```python
from build123d import *

# Parameters (mm, degrees)
SKETCH_R           = 62.5
SKETCH_R_2         = 7.75
SKETCH_R_3         = 1.5
SKETCH_R_4         = 5.5
SKETCH_R_5         = 4
PAD_DEPTH          = 10
SKETCH001_R        = 11.75
POCKET_DEPTH       = 3
FILLET_R           = 5
FILLET_FACE6_W     = 5
FILLET_FACE6_H     = 10
POCKET001_DEPTH    = 7
POCKET001_FACE39_W = 50
POCKET001_FACE39_H = 10
POCKET002_DEPTH    = 40.001
SKETCH002_R        = 1.5
POCKET003_DEPTH    = 10.001
POCKET004_DEPTH    = 10.001
CHAMFER_SIZE2      = 15
CHAMFER_SIZE       = 8.99
FILLET001_R        = 5


with BuildPart() as part:
    # Sketch → Pad (new body)
    with BuildSketch(Plane.XY):
        Polygon((-100, 100.02), (-100, -99.98), (55, -99.98), (55, -56.98), (60, -56.98), (60, -99.98), (100, -99.98), (100, 100.02), align=None)
        Circle(SKETCH_R, mode=Mode.SUBTRACT)
        with Locations((-82.5, -82.48)):
            Circle(SKETCH_R_2, mode=Mode.SUBTRACT)
        with Locations((-95, -94.98)):
            Circle(SKETCH_R_3, mode=Mode.SUBTRACT)
        with Locations((-95, -69.98)):
            Circle(SKETCH_R_3, mode=Mode.SUBTRACT)
        with Locations((-70, -69.98)):
            Circle(SKETCH_R_3, mode=Mode.SUBTRACT)
        with Locations((-70, -94.98)):
            Circle(SKETCH_R_3, mode=Mode.SUBTRACT)
        with Locations((-95, 95.02)):
            Circle(SKETCH_R_3, mode=Mode.SUBTRACT)
        with Locations((-70, 95.02)):
            Circle(SKETCH_R_3, mode=Mode.SUBTRACT)
        with Locations((-70, 70.02)):
            Circle(SKETCH_R_3, mode=Mode.SUBTRACT)
        with Locations((-95, 70.02)):
            Circle(SKETCH_R_3, mode=Mode.SUBTRACT)
        with Locations((-82.5, 82.52)):
            Circle(SKETCH_R_2, mode=Mode.SUBTRACT)
        with Locations((82.5, 82.52)):
            Circle(SKETCH_R_2, mode=Mode.SUBTRACT)
        with Locations((70, 95.02)):
            Circle(SKETCH_R_3, mode=Mode.SUBTRACT)
        with Locations((95, 95.02)):
            Circle(SKETCH_R_3, mode=Mode.SUBTRACT)
        with Locations((95, 70.02)):
            Circle(SKETCH_R_3, mode=Mode.SUBTRACT)
        with Locations((70, 70.02)):
            Circle(SKETCH_R_3, mode=Mode.SUBTRACT)
        with Locations((-85.5, 0)):
            Circle(SKETCH_R_4, mode=Mode.SUBTRACT)
        with Locations((-85.5, 8)):
            Circle(SKETCH_R_3, mode=Mode.SUBTRACT)
        with Locations((-77.5, 0)):
            Circle(SKETCH_R_3, mode=Mode.SUBTRACT)
        with Locations((-85.5, -8)):
            Circle(SKETCH_R_3, mode=Mode.SUBTRACT)
        with Locations((-93.5, 0)):
            Circle(SKETCH_R_3, mode=Mode.SUBTRACT)
        with Locations((0, 74.23)):
            Circle(SKETCH_R_5, mode=Mode.SUBTRACT)
        with Locations((68, -94.98)):
            Circle(SKETCH_R_3, mode=Mode.SUBTRACT)
        with Locations((93, -94.98)):
            Circle(SKETCH_R_3, mode=Mode.SUBTRACT)
    extrude(amount=PAD_DEPTH)

    # Sketch001 (on Face34 of Pad) → Pocket (cut)
    with BuildSketch(Plane.XY.offset(10)):
        with Locations((-85.5, 0)):
            Circle(SKETCH001_R)
    extrude(amount=-POCKET_DEPTH, mode=Mode.SUBTRACT)

    # Fillet
    fillet_edges = [part.edges().sort_by_distance(p)[0] for p in [
        (-100, -99.98, 5),
        (-100, 100.02, 5),
        (100, 100.02, 5),
        (100, -99.98, 5),
    ]]
    fillet(fillet_edges, radius=FILLET_R)

    # Fillet Face6 → Pocket001 (cut)
    with BuildSketch(Plane(origin=(57.5, -56.98, 5), x_dir=(-1, 0, 0), z_dir=(0, -1, 0))):
        Rectangle(FILLET_FACE6_W, FILLET_FACE6_H)
    extrude(amount=-POCKET001_DEPTH, mode=Mode.SUBTRACT)

    # Pocket001 Face39 → Pocket002 (cut, through all)
    with BuildSketch(Plane(origin=(60, -74.98, 5), x_dir=(0, 1, 0), z_dir=(-1, 0, 0))):
        Rectangle(POCKET001_FACE39_W, POCKET001_FACE39_H)
    extrude(amount=-POCKET002_DEPTH, mode=Mode.SUBTRACT)

    # Sketch002 (on Face32 of Pocket002) → Pocket003 (cut, through all)
    with BuildSketch(Plane.XY.offset(10)):
        with Locations((62.5, -45)):
            Circle(SKETCH002_R)
        with Locations((92.5, -45)):
            Circle(SKETCH002_R)
    extrude(amount=-POCKET003_DEPTH, mode=Mode.SUBTRACT)

    # Sketch003 (on Face35 of Pocket003) → Pocket004 (cut, through all)
    with BuildSketch(Plane.XY.offset(10)):
        Polygon((55, -58), (48, -58), (48, -67), (20, -67), (20, -100), (55, -100), align=None)
    extrude(amount=-POCKET004_DEPTH, mode=Mode.SUBTRACT)

    # Chamfer
    chamfer_edges = [part.edges().sort_by_distance(p)[0] for p in [
        (48, -67, 5),
    ]]
    chamfer_side = part.faces().sort_by_distance((48, -62.5, 5))[0]
    chamfer(chamfer_edges, length=CHAMFER_SIZE, length2=CHAMFER_SIZE2, reference=chamfer_side)

    # Fillet001
    fillet001_edges = [part.edges().sort_by_distance(p)[0] for p in [
        (20, -67, 5),
    ]]
    fillet(fillet001_edges, radius=FILLET001_R)


solid = part.part
```
For this review, take the finished solid that the model builds, in its own axes (mm). A direction names the side the tool comes from. Round coordinates to 2 decimals unless told otherwise and drop trailing zeros. Order: outer loops, then holes, each group sorted by start corner. A loop starts at its lowest first (then second) coordinate and runs counter-clockwise, first axis right, second up. Notation, with made-up numbers: (-34.75, 53.25) -> (-18.75, 53.25) arc R25 ccw to (-18.75, 82.25) -> close; hole circle Ø3 at (-33, 20). An arc over 180 degrees is marked (long way). Use a Markdown table: item, result.
Item 1: Take a section at C-C (z = 4.5). State how many separate pieces and enclosed holes the cut face has, plus the area to 3 significant figures.
Resolved:
| item | result |
|---|---|
| separate pieces | 1 |
| enclosed holes | 24 |
| area | 23,300 mm² |
Item 2: Take a section at B-B (x = 30). State the section outline as (y, z) points, plus the area to 3 significant figures.
Resolved:
| item | result |
|---|---|
| outline | (-67, 0) -> (-54.83, 0) -> (-54.83, 10) -> (-67, 10) -> close; (54.83, 0) -> (100.02, 0) -> (100.02, 10) -> (54.83, 10) -> close |
| area | 574 mm² |
Item 3: Take a section at A-A (y = 50). State the section outline as (x, z) points.
Resolved:
| item | result |
|---|---|
| outline | (-100, 0) -> (-37.5, 0) -> (-37.5, 10) -> (-100, 10) -> close; (37.5, 0) -> (100, 0) -> (100, 10) -> (37.5, 10) -> close |
Item 4: Draft analysis for pull direction Y (two halves, no side actions). For faces 1 (the flat face through (29, -67, 5)), 2 (the flat face through (-80, -2, 7)), 3 (the flat face through (100, 22, 5)), 4 (the flat face through (1, 100.02, 5)), state which applies: +Y half, -Y half, draft (parallel to the pull), parting line (faces both ways), or undercut.
Resolved:
| item | result |
|---|---|
| face 1 | -Y half |
| face 2 | undercut |
| face 3 | draft |
| face 4 | +Y half |
Item 5: Machinability: for faces 5 (the flat face through (20, -86, 5)), 6 (the cylindrical face through (-97.24, 0.52, 8.52)), 7 (the cylindrical face through (-98.57, -98.48, 5.07)), which of the approach directions +Z, -Z, +X, -X, +Y, -Y give a long, thin tool a straight path to every point of the face, cutting with its end or side? Answer none if there is none.
Resolved:
| item | result |
|---|---|
| face 5 | +Z, -Z, +X, -Y |
| face 6 | +Z |
| face 7 | +Z, -Z, -X, -Y |
Item 6: For pin 1 (3 mm diameter, centred on x = 66.5, z = 6.5, fed in from -Y); pin 2 (5 mm diameter, centred on x = -77.5, y = 0, fed in from +Z); pin 3 (5.5 mm diameter, centred on x = 52, z = 7, fed in from -Y), all flat-tipped, find the tip position at first contact; note any pin that passes through.
Resolved:
| item | result |
|---|---|
| pin 1 | stops at y = -49.98 |
| pin 2 | stops at z = 7 |
| pin 3 | stops at y = -58 |
Item 7: For line 1 along Y through (x, z) = (0, 7.5); line 2 along Y through (x, z) = (-70, 5); line 3 along X through (y, z) = (95.02, 5.5), list the stretches that pass through material, from the lowest coordinate up. Write a range as [from, to].
Resolved:
| item | result |
|---|---|
| line 1 | y = [-99.98, -62.5], [62.5, 70.23], [78.23, 100.02] |
| line 2 | y = [-99.98, -96.48], [-93.48, -71.48], [-68.48, 68.52], [71.52, 93.52], [96.52, 100.02] |
| line 3 | x = [-100, -96.5], [-93.5, -71.5], [-68.5, 68.5], [71.5, 93.5], [96.5, 100] |
